Work out the finished part from the listing and answer in its coordinate system (mm). A direction names the side the tool comes from. Round coordinates to 2 decimals unless told otherwise and drop trailing zeros. Write each loop counter-clockwise with the first axis right and the second up, starting at its lowest first coordinate (ties: lowest second). Pieces come first, ordered by that corner, then holes. Notation, with made-up numbers: (59, 42) -> (115, 42) arc R19 cw to (115, 76) -> close; hole circle Ø4 at (3.25, -30.75). An arc over 180 degrees is marked (long way). One line per question, with ' | ' between items. Start each with the question number.
```python
from build123d import *

# Parameters (mm, degrees)
EXTRUDE_1_DEPTH = 30
SKETCH_2_W      = 50
SKETCH_2_H      = 10
EXTRUDE_2_DEPTH = 50
HOLE_WIZARD_2_D = 5.2
HOLE_WIZARD_3_D = 9
SKETCH_17_R     = 2.45
EXTRUDE_6_DEPTH = 4
HOLE_WIZARD_5_D = 3
EXTRUDE_7_DEPTH = 50


with BuildPart() as part:
    # 草图1 → 凸台-拉伸1 (new body)
    with BuildSketch(Plane.XY):
        Polygon((13.1, -5.375), (13.1, -25.375), (10.1, -25.375), (10.1, -5.375), (-10.1, -5.375), (-10.1, -25.375), (-13.1, -25.375), (-13.1, -5.375), (-25, -5.375), (-25, 5.375), (25, 5.375), (25, -5.375), align=None)
    extrude(amount=EXTRUDE_1_DEPTH)

    # 草图2 → 凸台-拉伸2 (add)
    with BuildSketch(Plane(origin=(0, 5.375, 0), x_dir=(1, 0, 0), z_dir=(0, 1, 0))):
        with Locations((0, -15)):
            Rectangle(SKETCH_2_W, SKETCH_2_H)
    extrude(amount=EXTRUDE_2_DEPTH)

    # 孔2 (through all)
    with Locations(Plane.ZY.offset(13.1)):
        with Locations((7, -15.375), (23, -15.375)):
            Hole(HOLE_WIZARD_2_D / 2)

    # 孔3 (through all)
    with Locations(Plane(origin=(0, 0, 10), x_dir=(-1, 0, 0), z_dir=(0, 0, -1))):
        with Locations((0, 35.625)):
            Hole(HOLE_WIZARD_3_D / 2)

    # 草图17 → 凸台-拉伸6 (add)
    with BuildSketch(Plane(origin=(0, 0, 10), x_dir=(-1, 0, 0), z_dir=(0, 0, -1))):
        with Locations(Location((18.25, 35.625, 0), (0, 0, 180))):
            Circle(SKETCH_17_R)
        with Locations(Location((-18.25, 35.625, 0), (0, 0, 180))):
            Circle(SKETCH_17_R)
    extrude(amount=EXTRUDE_6_DEPTH)

    # 孔5 (through all)
    with Locations(Plane(origin=(0, 0, 6), x_dir=(-1, 0, 0), z_dir=(0, 0, -1))):
        with Locations((18.25, 35.625), (-18.25, 35.625)):
            Hole(HOLE_WIZARD_5_D / 2)

    # 草图20 → 凸台-拉伸7 (add)
    with BuildSketch(Plane.ZY.offset(25)):
        Polygon((20, 18.375), (30, 5.375), (20, 5.375), align=None)
        Polygon((10, 18.375), (0, 5.375), (10, 5.375), align=None)
    extrude(amount=-EXTRUDE_7_DEPTH)


solid = part.part
```
(1) A cutting plane is placed at A-A, the plane x = 18.25. Determine the outline of the cut face in (y, z) (3 decimals), then the cut area to 3 significant figures.
(2) For faces 5 (the cylindrical face through (17.9, 33.2, 8)), 6 (the flat face through (0, 41, 20)), 7 (the flat face through (-13.1, -16, 15)), determine the directions among +Z, -Z, +X, -X, +Y, -Y from which every point of the face is accessible in a straight line to the end or side of a thin tool.
(3) A cutting plane is placed at B-B, the plane z = 7.25. Determine the outline of the cut face in (x, y) (3 decimals), then the cut area to 3 significant figures.
(4) Consider L1, parallel to Y at x = 0, z = 16 (3 decimals); L2, parallel to Y at x = 18.25, z = 12 (3 decimals); L3, parallel to Z at x = 0, y = 28. Determine where each line is inside the solid, lowest interval first.
(5) The mould has two halves that part along Z. Classify faces 1 (the cylindrical face through (-11.58, -16.37, 20.6)), 2 (the cylindrical face through (11.62, -16.37, 4.6)), 3 (the cylindrical face through (-0.976, 31.232, 15.07)), 4 (the flat face through (-16.65, 36.14, 6)): +Z half, -Z half, draft (parallel to the pull), parting line (faces both ways), or undercut.
(6) A cutting plane is placed at D-D, the plane z = 23. Determine the outline of the cut face in (x, y) (3 decimals).
(7) A cutting plane is placed at C-C, the plane y = -11. Determine the outline of the cut face in (x, z).
(8) Given pin 1 Ø5 at (x, y) = (18.25, 35.625) entering from +Z; pin 2 Ø7 at (y, z) = (-15.375, 23) entering from -X; pin 3 Ø6 at (x, z) = (-16, 15) entering from -Y (3 decimals); pin 4 Ø10.5 at (x, y) = (0, 35.625) entering from -Z, each flat-ended and moving along its own axis, determine where each tip first touches the part or whether it passes through.
Returned:
1) outline: (-5.375, 0) -> (5.375, 0) -> (18.375, 10) -> (33.175, 10) -> (33.175, 6) -> (34.125, 6) -> (34.125, 20) -> (18.375, 20) -> (5.375, 30) -> (-5.375, 30) -> close; (37.125, 6) -> (38.075, 6) -> (38.075, 10) -> (55.375, 10) -> (55.375, 20) -> (37.125, 20) -> close | area: 930 mm2
2) face 5: -Z | face 6: +Z, +X, -X, +Y | face 7: +Z, -Z, -X, -Y
3) outline: (-25, -5.375) -> (-13.1, -5.375) -> (-13.1, -12.787) -> (-10.1, -12.787) -> (-10.1, -5.375) -> (10.1, -5.375) -> (10.1, -12.787) -> (13.1, -12.787) -> (13.1, -5.375) -> (25, -5.375) -> (25, 14.8) -> (-25, 14.8) -> close; circle Ø4.9 at (-18.25, 35.625); (-13.1, -25.375) -> (-10.1, -25.375) -> (-10.1, -17.963) -> (-13.1, -17.963) -> close; (10.1, -25.375) -> (13.1, -25.375) -> (13.1, -17.963) -> (10.1, -17.963) -> close; circle Ø4.9 at (18.25, 35.625); hole circle Ø3 at (-18.25, 35.625); hole circle Ø3 at (18.25, 35.625) | area: 1,120 mm2
4) L1: -5.375 to 31.125, 40.125 to 55.375 | L2: -5.375 to 34.125, 37.125 to 55.375 | L3: 10 to 20
5) face 1: undercut | face 2: undercut | face 3: draft | face 4: -Z half
6) outline: (-25, -5.375) -> (-13.1, -5.375) -> (-13.1, -12.775) -> (-10.1, -12.775) -> (-10.1, -5.375) -> (10.1, -5.375) -> (10.1, -12.775) -> (13.1, -12.775) -> (13.1, -5.375) -> (25, -5.375) -> (25, 14.475) -> (-25, 14.475) -> close; (-13.1, -25.375) -> (-10.1, -25.375) -> (-10.1, -17.975) -> (-13.1, -17.975) -> close; (10.1, -25.375) -> (13.1, -25.375) -> (13.1, -17.975) -> (10.1, -17.975) -> close
7) outline: (-13.1, 0) -> (-10.1, 0) -> (-10.1, 30) -> (-13.1, 30) -> close; (10.1, 0) -> (13.1, 0) -> (13.1, 30) -> (10.1, 30) -> close
8) pin 1: z = 20 | pin 2: x = -13.1 | pin 3: y = -25.375 | pin 4: z = 10
